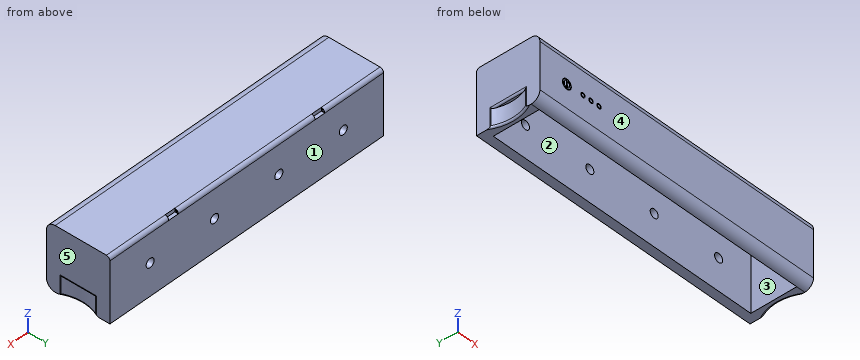
from build123d import *

# Parameters (mm, degrees)
SKETCH1_W           = 85
SKETCH1_H           = 18.1
BOSS_EXTRUDE1_DEPTH = 18.1
SKETCH2_W           = 80
SKETCH2_H           = 13.1
CUT_EXTRUDE1_DEPTH  = 17.5
SKETCH3_R           = 1.25
CUT_EXTRUDE2_DEPTH  = 2.5
SKETCH4_W           = 3
SKETCH4_H           = 1
CUT_EXTRUDE4_DEPTH  = 1
BOSS_EXTRUDE3_DEPTH = 1
SKETCH5_R           = 0.25
CUT_EXTRUDE5_DEPTH  = 0.25
CUT_EXTRUDE6_START  = -0.25
SKETCH6_R           = 0.25
CUT_EXTRUDE6_DEPTH  = 0.25
CUT_EXTRUDE7_START  = -0.25
SKETCH7_R           = 0.25
CUT_EXTRUDE7_DEPTH  = 0.25
SKETCH8_R           = 0.25
CUT_EXTRUDE8_DEPTH  = 0.25
CUT_EXTRUDE9_REACH  = 89.376
SKETCH13_R          = 1.390804474
SKETCH13_R_2        = 0.659370612
SKETCH13_R_3        = 0.42561601
CUT_EXTRUDE10_DEPTH = 0.5
CUT_EXTRUDE11_DEPTH = 5
FILLET1_R           = 0.5
CUT_EXTRUDE12_START = -85
CUT_EXTRUDE12_DEPTH = 85


with BuildPart() as part:
    # Sketch1 → Boss-Extrude1 (new body)
    with BuildSketch(Plane.XY):
        Rectangle(SKETCH1_W, SKETCH1_H)
    extrude(amount=BOSS_EXTRUDE1_DEPTH)

    # Sketch2 → Cut-Extrude1 (cut)
    with BuildSketch(Plane(origin=(0, 0, 0), x_dir=(-1, 0, 0), z_dir=(0, 0, -1))):
        Rectangle(SKETCH2_W, SKETCH2_H)
    extrude(amount=-CUT_EXTRUDE1_DEPTH, mode=Mode.SUBTRACT)

    # Sketch3 → Cut-Extrude2 (cut)
    with BuildSketch(Plane(origin=(0, 9.05, 0), x_dir=(1, 0, 0), z_dir=(0, 1, 0))):
        with Locations(Location((-30, -9.05, 0), (0, 0, 180))):
            Circle(SKETCH3_R)
        with Locations(Location((-10, -9.05, 0), (0, 0, 180))):
            Circle(SKETCH3_R)
        with Locations(Location((10, -9.05, 0), (0, 0, 180))):
            Circle(SKETCH3_R)
        with Locations(Location((30, -9.05, 0), (0, 0, 180))):
            Circle(SKETCH3_R)
    extrude(amount=-CUT_EXTRUDE2_DEPTH, mode=Mode.SUBTRACT)

    # Sketch4 → Cut-Extrude4 (cut)
    with BuildSketch(Plane.XY.offset(18.1)):
        with Locations((-22.75, 8.55)):
            Rectangle(SKETCH4_W, SKETCH4_H)
        with Locations((22.75, 8.55)):
            Rectangle(SKETCH4_W, SKETCH4_H)
    extrude(amount=-CUT_EXTRUDE4_DEPTH, mode=Mode.SUBTRACT)

    # Sketch11 → Boss-Extrude3 (add)
    with BuildSketch(Plane.XY.offset(18.1)):
        Polygon((-24.25, 8.05), (-24.25, 9.05), (-42.5, 9.05), (-42.5, -9.05), (42.5, -9.05), (42.5, 9.05), (24.25, 9.05), (24.25, 8.05), (21.25, 8.05), (21.25, 9.05), (-21.25, 9.05), (-21.25, 8.05), align=None)
    extrude(amount=-BOSS_EXTRUDE3_DEPTH)

    # Sketch5 → Cut-Extrude5 (cut)
    with BuildSketch(Plane(origin=(-24.25, 0, 0), x_dir=(0, 0, -1), z_dir=(1, 0, 0))):
        with Locations((-17.6, 8.55)):
            Circle(SKETCH5_R)
    extrude(amount=-CUT_EXTRUDE5_DEPTH, mode=Mode.SUBTRACT)

    # Sketch6 → Cut-Extrude6 (cut)
    with BuildSketch(Plane.ZY.offset(21.25).offset(CUT_EXTRUDE6_START)):
        with Locations(Location((17.6, 8.55, 0), (0, 0, 180))):
            Circle(SKETCH6_R)
    extrude(amount=CUT_EXTRUDE6_DEPTH, mode=Mode.SUBTRACT)

    # Sketch7 → Cut-Extrude7 (cut)
    with BuildSketch(Plane.ZY.offset(-24.25).offset(CUT_EXTRUDE7_START)):
        with Locations(Location((17.6, 8.55, 0), (0, 0, 180))):
            Circle(SKETCH7_R)
    extrude(amount=CUT_EXTRUDE7_DEPTH, mode=Mode.SUBTRACT)

    # Sketch8 → Cut-Extrude8 (cut)
    with BuildSketch(Plane(origin=(21.25, 0, 0), x_dir=(0, 0, -1), z_dir=(1, 0, 0))):
        with Locations((-17.6, 8.55)):
            Circle(SKETCH8_R)
    extrude(amount=-CUT_EXTRUDE8_DEPTH, mode=Mode.SUBTRACT)

    # Cut-Extrude9: up to this face of the body (flat: up to its plane)
    cut_extrude9_end = Plane(part.part.faces().sort_by_distance((-42.5, 0, 9.05))[0])
    # Sketch12 → Cut-Extrude9 (cut, up to the picked face)
    with BuildSketch(Plane(origin=(42.5, 0, 0), x_dir=(0, 0, -1), z_dir=(1, 0, 0)), mode=Mode.PRIVATE) as cut_extrude9_sk1:
        with BuildLine():
            Line((-18.1, -6.55), (-18.1, -9.05))
            Line((-18.1, -9.05), (-15.6, -9.05))
            ThreePointArc((-15.6, -9.05), (-17.367766953, -8.317766953), (-18.1, -6.55))
        make_face()
    cut_extrude9_tool1 = split(extrude(cut_extrude9_sk1.sketch, amount=-CUT_EXTRUDE9_REACH, mode=Mode.PRIVATE), bisect_by=cut_extrude9_end, keep=Keep.BOTH, mode=Mode.PRIVATE)
    # Sketch12 → Cut-Extrude9 (cut, up to the picked face)
    with BuildSketch(Plane(origin=(42.5, 0, 0), x_dir=(0, 0, -1), z_dir=(1, 0, 0)), mode=Mode.PRIVATE) as cut_extrude9_sk2:
        with BuildLine():
            Line((-2.5, -9.05), (0, -9.05))
            Line((0, -9.05), (0, -6.55))
            ThreePointArc((0, -6.55), (-0.732233047, -8.317766953), (-2.5, -9.05))
        make_face()
    cut_extrude9_tool2 = split(extrude(cut_extrude9_sk2.sketch, amount=-CUT_EXTRUDE9_REACH, mode=Mode.PRIVATE), bisect_by=cut_extrude9_end, keep=Keep.BOTH, mode=Mode.PRIVATE)
    add(cut_extrude9_tool1.solids().sort_by(Axis((42.5, -8.49158, 17.54158), (-1, 0, 0)))[0], mode=Mode.SUBTRACT)
    add(cut_extrude9_tool2.solids().sort_by(Axis((42.5, -8.49158, 0.55842), (-1, 0, 0)))[0], mode=Mode.SUBTRACT)

    # Sketch13 → Cut-Extrude10 (cut)
    # profile 1 of 4: a face of its own
    with BuildSketch(Plane.XZ.offset(9.05)):
        with Locations((-34.135654856, 9.05)):
            Circle(SKETCH13_R)
        with BuildLine():
            Line((-34.009203979, 10.17572082), (-34.009203979, 8.391358435))
            ThreePointArc((-34.009203979, 8.391358435), (-34.135654856, 8.264907558), (-34.262105734, 8.391358435))
            Line((-34.262105734, 8.391358435), (-34.262105734, 10.17572082))
            ThreePointArc((-34.262105734, 10.17572082), (-34.135654856, 10.302171697), (-34.009203979, 10.17572082))
        make_face(mode=Mode.SUBTRACT)
        with BuildLine():
            ThreePointArc((-34.868750994, 10.048689821), (-34.135654856, 7.811124984), (-33.402558718, 10.048689821))
            ThreePointArc((-33.402558718, 10.048689821), (-33.657371419, 10.009610716), (-33.618292315, 9.754798016))
            ThreePointArc((-33.618292315, 9.754798016), (-34.135654856, 8.175697855), (-34.653017397, 9.754798016))
            ThreePointArc((-34.653017397, 9.754798016), (-34.613938293, 10.009610716), (-34.868750994, 10.048689821))
        make_face(mode=Mode.SUBTRACT)
    # profile 2 of 4: a face of its own
    with BuildSketch(Plane.XZ.offset(9.05)):
        with Locations((-29.135654856, 9.05)):
            Circle(SKETCH13_R_2)
        with Locations((-29.135654856, 9.05)):
            Circle(SKETCH13_R_3, mode=Mode.SUBTRACT)
    # profile 3 of 4: a face of its own
    with BuildSketch(Plane.XZ.offset(9.05)):
        with Locations((-26.635654856, 9.05)):
            Circle(SKETCH13_R_2)
        with Locations((-26.635654856, 9.05)):
            Circle(SKETCH13_R_3, mode=Mode.SUBTRACT)
    # profile 4 of 4: a face of its own
    with BuildSketch(Plane.XZ.offset(9.05)):
        with Locations((-24.135654856, 9.05)):
            Circle(SKETCH13_R_2)
        with Locations((-24.135654856, 9.05)):
            Circle(SKETCH13_R_3, mode=Mode.SUBTRACT)
    extrude(amount=-CUT_EXTRUDE10_DEPTH, mode=Mode.SUBTRACT)

    # Sketch16 → Cut-Extrude11 (cut)
    with BuildSketch(Plane(origin=(0, 0, 0), x_dir=(-1, 0, 0), z_dir=(0, 0, -1))):
        with BuildLine():
            Line((-42.5, -5.059421515), (-42.5, 5.059421515))
            ThreePointArc((-42.5, 5.059421515), (-41.365768493, 0), (-42.5, -5.059421515))
        make_face()
        with BuildLine():
            Line((42.5, -5.059421515), (42.5, 5.059421515))
            ThreePointArc((42.5, 5.059421515), (41.365768493, 0), (42.5, -5.059421515))
        make_face()
    extrude(amount=-CUT_EXTRUDE11_DEPTH, mode=Mode.SUBTRACT)

    # Fillet1
    fillet1_edges = [part.edges().sort_by_distance(p)[0] for p in [
        (-42.5, -5.059421515, 2.5),
        (-42.5, 0, 5),
        (-42.5, 5.059421515, 2.5),
        (-41.365768493, 0, 0),
        (42.5, 5.059421515, 2.5),
        (42.5, 0, 5),
        (42.5, -5.059421515, 2.5),
        (41.365768493, 0, 0),
    ]]
    fillet(fillet1_edges, radius=FILLET1_R)

    # Sketch17 → Cut-Extrude12 (cut)
    with BuildSketch(Plane(origin=(42.5, 0, 0), x_dir=(0, 0, -1), z_dir=(1, 0, 0)).offset(CUT_EXTRUDE12_START)):
        with BuildLine():
            Line((-18.1, 8.05), (-18.1, 9.05))
            Line((-18.1, 9.05), (-17.1, 9.05))
            ThreePointArc((-17.1, 9.05), (-17.807106781, 8.757106781), (-18.1, 8.05))
        make_face()
    extrude(amount=CUT_EXTRUDE12_DEPTH, mode=Mode.SUBTRACT)


solid = part.part
Source: CAD feature listing. Evaluate the final solid. Frame: model axes, mm. Face numbers are marked on the shaded views. A direction names the side the tool comes from. Give positions to 0.01 mm unless a question says otherwise; leave off trailing zeros. Write each loop counter-clockwise with the first axis right and the second up, starting at its lowest first coordinate (ties: lowest second). Pieces come first, ordered by that corner, then holes. Notation, with made-up numbers: (47.25, 64) -> (103.25, 64) arc R20 cw to (103.25, 98) -> close; hole circle Ø5 at (45.25, -30). An arc over 180 degrees is marked (long way). Return JSON: item names as keys, results as strings. Group by question number.
1. Access query for the marked faces 1 and 2. Directions: +Z, -Z, +X, -X, +Y, -Y. A direction counts if a zero-diameter tool reaches every point of the face in a straight line with its end or side. Return the directions, or none.
2. Material intervals for line 1 (X direction, y = 6, z = 7.75); line 2 (Y direction, x = -10, z = 13.25); line 3 (Z direction, x = -30, y = 8.05), sorted ascending. Write a range as from..to.
3. Pin query (flat end, axial travel): pin 1 Ø0.5 at (x, y) = (22, 8.5) entering from +Z; pin 2 Ø3 at (y, z) = (-0.5, 3) entering from +X; pin 3 Ø1.1 at (x, z) = (22.5, 18) entering from +Y. Return the tip coordinate at first contact, or that it passes through.
4. Mould query, pull axis X, two halves, no side actions, for the marked faces 3, 4 and 5. Classes: +X half, -X half, draft (parallel to the pull), parting line (faces both ways), or undercut.
5. Section A-A, the plane x = 10. Output: boundary loops of the cut face in (y, z).
6. Section B-B, the plane z = 12.75. Output: boundary loops of the cut face in (x, y).
Determined:
{
 "1": {"face 1": "+Z, -Z, +X, -X, +Y", "face 2": "-Z"},
 "2": {"line 1": "x = -42.5..-40, 40..42.5", "line 2": "y = -9.05..-6.55, 6.55..9.05", "line 3": "z = 0..7.8, 10.3..18.1"},
 "3": {"pin 1": "stops at z = 17.1", "pin 2": "stops at x = 41.54", "pin 3": "stops at y = 8.05"},
 "4": {"face 3": "undercut", "face 4": "draft", "face 5": "+X half"},
 "5": {"outline": "(-9.05, 2.5) arc R2.5 ccw to (-6.55, 0) -> (-6.55, 17.1) -> (6.55, 17.1) -> (6.55, 10.3) -> (9.05, 10.3) -> (9.05, 17.1) arc R1 ccw to (8.05, 18.1) -> (-6.55, 18.1) arc R2.5 ccw to (-9.05, 15.6) -> close; (6.55, 0) -> (9.05, 0) -> (9.05, 7.8) -> (6.55, 7.8) -> close"},
 "6": {"outline": "(-42.5, -9.05) -> (42.5, -9.05) -> (42.5, 9.05) -> (-42.5, 9.05) -> close; hole (-40, -6.55) -> (40, -6.55) -> (40, 6.55) -> (-40, 6.55) -> close"}
}
